Source: CAD feature listing. Evaluate the final solid. Frame: model axes, mm. Coordinates: 2 decimals unless noted, no trailing zeros. Write each loop counter-clockwise with the first axis right and the second up, starting at its lowest first coordinate (ties: lowest second). Pieces come first, ordered by that corner, then holes. Notation, with made-up numbers: M -3,45.5 L 18,45.5 A29 ccw 18,67.5 Z; hole C 41.5,65.5 d9. An arc over 180 degrees is marked long. One line per item, written item: value. Start each with the question number.
Item 1: Cut plane A-A, the plane x = 43. Output: boundary loops of the cut face in (y, z).
Item 2: Pin query (flat end, axial travel): P1, Ø1, axis at y = -8.5, z = 2.5, coming from the -X side; P2, Ø1, axis at x = -60, z = 2.5, coming from the -Y side; P3, Ø1.6, axis at y = 4.76, z = 3.18, coming from the -X side; P4, Ø3, axis at x = -15.88, y = -4.76, coming from the -Z side. Return the tip coordinate at first contact, or that it passes through.
Item 3: Ray query, L1, parallel to X at y = 0, z = 3 (3 decimals); L2, parallel to X at y = -11.5, z = 0.5; L3, parallel to X at y = -9.5, z = 2.75 (3 decimals). Return the intervals inside material, ascending. Write a range as from..to.
```python
from build123d import *

# Parameters (mm, degrees)
BOSS_EXTRUDE1_DEPTH                               = 6.35
TAP_DRILL_FOR_6_32_TAP1_AT_2_COUNT                = 2
TAP_DRILL_FOR_6_32_TAP1_AT_2_PITCH                = 9.525
SKETCH7_W                                         = 6.35
SKETCH7_H                                         = 1.5875
CUT_EXTRUDE1_DEPTH                                = 91.02678768
SKETCH10_W                                        = 6.35
SKETCH10_H                                        = 1.5875
SKETCH10_W_2                                      = 33.02
SKETCH10_H_2                                      = 22.225
CUT_EXTRUDE5_DEPTH                                = 91.02678768
CSK_FOR_6_FLAT_HEAD_MACHINE_SCREW_100_D           = 3.7973
CSK_FOR_6_FLAT_HEAD_MACHINE_SCREW_100_CSINK_D     = 7.0866
CSK_FOR_6_FLAT_HEAD_MACHINE_SCREW_100_CSINK_ANGLE = 100
CSK_FOR_6_FLAT_HEAD_MACHINE_SCREW_2_D             = 3.7973
CSK_FOR_6_FLAT_HEAD_MACHINE_SCREW_2_CSINK_D       = 7.0866
CSK_FOR_6_FLAT_HEAD_MACHINE_SCREW_2_CSINK_ANGLE   = 100


with BuildPart() as part:
    # Sketch1 → Boss-Extrude1 (new body)
    with BuildSketch(Plane.XY):
        Polygon((-88.9, 12.7), (88.9, 12.7), (88.9, 11.1125), (82.55, 11.1125), (82.55, -11.1125), (88.9, -11.1125), (88.9, -12.7), (-88.9, -12.7), (-88.9, -11.1125), (-82.55, -11.1125), (-82.55, 11.1125), (-88.9, 11.1125), align=None)
    extrude(amount=BOSS_EXTRUDE1_DEPTH)

    # Sketch4 → Tap Drill for #6-32 Tap1 (revolve, cut)
    with BuildSketch(Plane(origin=(-82.55, 4.7625, 3.175), x_dir=(0, 0, 1), z_dir=(0, 1, 0))):
        Polygon((0, 0), (0, 13.51269403), (1.35255, 12.7), (1.35255, 0), align=None)
    tap_drill_for_6_32_tap1 = revolve(axis=Axis((-88.9, 4.7625, 3.175), (1, 0, 0)), mode=Mode.SUBTRACT)

    # Tap Drill for #6-32 Tap1 at 2: Tap Drill for #6-32 Tap1 ×2
    with Locations(*[(0, -i * TAP_DRILL_FOR_6_32_TAP1_AT_2_PITCH, 0) for i in range(1, TAP_DRILL_FOR_6_32_TAP1_AT_2_COUNT)]):
        add(tap_drill_for_6_32_tap1, mode=Mode.SUBTRACT)

    # Mirror1: Tap Drill for #6-32 Tap1 across plane
    add(tap_drill_for_6_32_tap1.mirror(Plane(origin=(0, 0, 0), x_dir=(0, 0, 1), z_dir=(1, 0, 0))), mode=Mode.SUBTRACT)

    # Mirror1 copy 1 sketch → Mirror1 copy 1 (revolve, cut)
    with BuildSketch(Plane(origin=(82.55, -4.7625, 3.175), x_dir=(0, 0, 1), z_dir=(0, 1, 0))):
        Polygon((0, 0), (0, -13.51269403), (1.35255, -12.7), (1.35255, 0), align=None)
    revolve(axis=Axis((88.9, -4.7625, 3.175), (1, 0, 0)), mode=Mode.SUBTRACT)

    # Sketch5 → Tap Drill for #6-32 Tap2 (revolve, cut)
    with BuildSketch(Plane(origin=(-73.289583418, 12.7, 3.175), x_dir=(0, 0, 1), z_dir=(1, 0, 0))):
        Polygon((0, 0), (0, 7.16269403), (1.35255, 6.35), (1.35255, 0), align=None)
    tap_drill_for_6_32_tap2 = revolve(axis=Axis((-73.289583418, 19.05, 3.175), (0, -1, 0)), mode=Mode.SUBTRACT)

    # Mirror2: Tap Drill for #6-32 Tap2 across plane
    add(tap_drill_for_6_32_tap2.mirror(Plane(origin=(0, 0, 0), x_dir=(0, 0, 1), z_dir=(1, 0, 0))), mode=Mode.SUBTRACT)

    # Mirror3: Tap Drill for #6-32 Tap2 across plane
    add(tap_drill_for_6_32_tap2.mirror(Plane(origin=(0, 0, 0), x_dir=(0, 0, 1), z_dir=(0, -1, 0))), mode=Mode.SUBTRACT)

    # Mirror3 copy 1 sketch → Mirror3 copy 1 (revolve, cut)
    with BuildSketch(Plane(origin=(73.289583418, -12.7, 3.175), x_dir=(0, 0, 1), z_dir=(-1, 0, 0))):
        Polygon((0, 0), (0, 7.16269403), (1.35255, 6.35), (1.35255, 0), align=None)
    revolve(axis=Axis((73.289583418, -19.05, 3.175), (0, 1, 0)), mode=Mode.SUBTRACT)

    # Sketch7 → Cut-Extrude1 (cut, through all)
    with BuildSketch(Plane.XY.offset(6.35)):
        with Locations((-61.595, 11.90625)):
            Rectangle(SKETCH7_W, SKETCH7_H)
        with Locations((-61.595, -11.90625)):
            Rectangle(SKETCH7_W, SKETCH7_H)
        with Locations((61.595, -11.90625)):
            Rectangle(SKETCH7_W, SKETCH7_H)
        with Locations((61.595, 11.90625)):
            Rectangle(SKETCH7_W, SKETCH7_H)
    extrude(amount=-CUT_EXTRUDE1_DEPTH, mode=Mode.SUBTRACT)

    # Sketch10 → Cut-Extrude5 (cut, through all)
    with BuildSketch(Plane(origin=(0, 0, 0), x_dir=(-1, 0, 0), z_dir=(0, 0, -1))):
        with Locations((-15.875, 11.90625)):
            Rectangle(SKETCH10_W, SKETCH10_H)
        with Locations((15.875, 11.90625)):
            Rectangle(SKETCH10_W, SKETCH10_H)
        with Locations((-15.875, -11.90625)):
            Rectangle(SKETCH10_W, SKETCH10_H)
        with Locations((15.875, -11.90625)):
            Rectangle(SKETCH10_W, SKETCH10_H)
        with Locations((-38.735, 0)):
            Rectangle(SKETCH10_W_2, SKETCH10_H_2)
        with Locations((38.735, 0)):
            Rectangle(SKETCH10_W_2, SKETCH10_H_2)
    extrude(amount=-CUT_EXTRUDE5_DEPTH, mode=Mode.SUBTRACT)

    # CSK for _6 Flat Head Machine Screw _100 (through all)
    with Locations(Plane.XY.offset(6.35)):
        with Locations((-61.595, 4.7625), (-61.595, -4.7625)):
            csk_for_6_flat_head_machine_screw_100 = CounterSinkHole(CSK_FOR_6_FLAT_HEAD_MACHINE_SCREW_100_D / 2, CSK_FOR_6_FLAT_HEAD_MACHINE_SCREW_100_CSINK_D / 2, counter_sink_angle=CSK_FOR_6_FLAT_HEAD_MACHINE_SCREW_100_CSINK_ANGLE)

    # CSK for _6 Flat Head Machine Screw _ 2 (through all)
    with Locations(Plane(origin=(0, 0, 0), x_dir=(-1, 0, 0), z_dir=(0, 0, -1))):
        with Locations((15.875, 4.7625), (15.875, -4.7625)):
            csk_for_6_flat_head_machine_screw_2 = CounterSinkHole(CSK_FOR_6_FLAT_HEAD_MACHINE_SCREW_2_D / 2, CSK_FOR_6_FLAT_HEAD_MACHINE_SCREW_2_CSINK_D / 2, counter_sink_angle=CSK_FOR_6_FLAT_HEAD_MACHINE_SCREW_2_CSINK_ANGLE)

    # Mirror5: CSK for _6 Flat Head Machine Screw _100, CSK for _6 Flat Head Machine Screw _ 2 across plane
    add(csk_for_6_flat_head_machine_screw_100.mirror(Plane(origin=(0, 0, 0), x_dir=(0, 0, 1), z_dir=(1, 0, 0))), mode=Mode.SUBTRACT)
    add(csk_for_6_flat_head_machine_screw_2.mirror(Plane(origin=(0, 0, 0), x_dir=(0, 0, 1), z_dir=(1, 0, 0))), mode=Mode.SUBTRACT)


solid = part.part
```
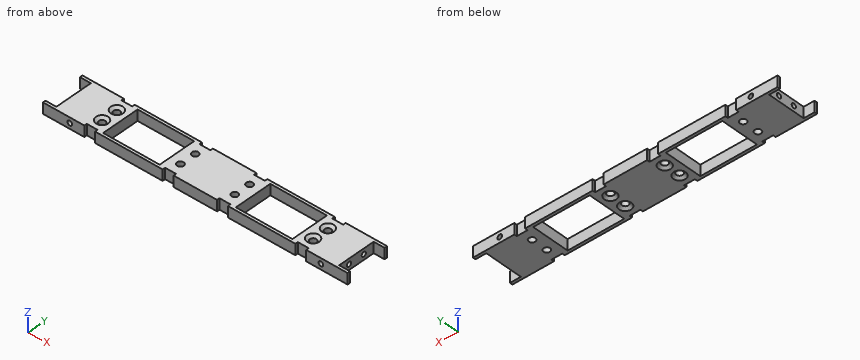
From the geometry:
1. outline: M -12.7,0 L -11.11,0 L -11.11,6.35 L -12.7,6.35 Z; M 11.11,0 L 12.7,0 L 12.7,6.35 L 11.11,6.35 Z
2. P1: stops at x = -82.55
2. P2: stops at y = -11.11
2. P3: stops at x = -69.52
2. P4: passes through
3. L1: x = -82.55..-55.245, -22.225..22.225, 55.245..82.55
3. L2: x = -88.9..-64.77, -58.42..-19.05, -12.7..12.7, 19.05..58.42, 64.77..88.9
3. L3: x = -82.55..-74.574, -72.006..-55.245, -22.225..22.225, 55.245..72.006, 74.574..82.55
